Verification items for the finished model (mm, model axes). A direction names the side the tool comes from. Give positions to 0.01 mm unless a question says otherwise; leave off trailing zeros. Loops run counter-clockwise (first coordinate to the right, second up) from the corner with the lowest first, then second, coordinate; pieces in that order, holes last. Notation, with made-up numbers: (65.25, -21.75) -> (109.25, -21.75) arc R13 cw to (109.25, -17.75) -> close; hole circle Ø8 at (84.25, 73.5). An arc over 180 degrees is marked (long way). Answer in a Markdown table with one row per item. Add a question column.
Q1. Material ranges on probe 1 along Y at (x, z) = (-8.5, -10.5); probe 2 along Z at (x, y) = (-3.75, 3.75); probe 3 along Z at (x, y) = (13.25, 1.5), recorded low to high.
Q2. Section check C-C on x = -4. Enter the section's corners in (y, z), and give its area (3 significant figures).
Q3. Release check for a two-part mould opening along Z. For faces 1 (the face through (8, 1.8, -9)), 2 (the face through (0, 2.54, 8)), 3 (the face through (-6, 1, 7.562)) record: pulls with the +Z half, pulls with the -Z half, needs draft (parallel to the pull), parting line crosses it, or undercut.
Q4. Gauge pin test, flat ends, axial feed: P1, Ø1.5, axis at x = 11, y = 1.5, coming from the -Z side; P2, Ø2, axis at y = 1, z = 7.5, coming from the +X side; P3, Ø2, axis at x = -8.5, y = 0.5, coming from the +Z side; P4, Ø1, axis at x = -2.5, z = 9, coming from the +Y side. Record the tip position at first contact, or that the pin passes through.
Q5. Section check D-D on y = 0.75. Enter the section's corners in (x, z).
Q6. Section check B-B on z = -16. Enter the section's corners in (x, y).
Q7. Section check A-A on y = 3. Enter the section's corners in (x, z), and give its area (3 significant figures).
Q8. Set-up check for faces 4 (the face through (0, 6.88, -17)), 5 (the face through (11, 1, 5)), 6 (the face through (11, 1, -11)): record each of +Z, -Z, +X, -X, +Y, -Y from which the full face is reachable in a straight line by a thin tool's end or side.
```python
from build123d import *

# Parameters (mm, degrees)
SKETCH1_W           = 22
SKETCH1_H           = 28.216692514
BOSS_EXTRUDE1_DEPTH = 1.8
BOSS_EXTRUDE4_DEPTH = 2.54
SKETCH2_W           = 5.08
SKETCH2_H           = 5.08
BOSS_EXTRUDE2_DEPTH = 0.79375
BOSS_EXTRUDE3_START = -1.8
SKETCH3_W           = 7.62
SKETCH3_H           = 2.54
SKETCH3_W_2         = 20.32
SKETCH3_H_2         = 5.08
BOSS_EXTRUDE3_DEPTH = 5.08


with BuildPart() as part:
    # Sketch1 → Boss-Extrude1 (new body)
    with BuildSketch(Plane(origin=(0, 0, 0), x_dir=(1, 0, 0), z_dir=(0, 1, 0))):
        with Locations((0, 6.545846257)):
            Rectangle(SKETCH1_W, SKETCH1_H)
    extrude(amount=BOSS_EXTRUDE1_DEPTH)

    # Sketch4 → Boss-Extrude4 (add)
    with BuildSketch(Plane(origin=(0, 0, 0), x_dir=(1, 0, 0), z_dir=(0, 1, 0))):
        Polygon((-14.2875, -1.5875), (-1.5875, -1.5875), (-1.5875, -14.2875), (1.5875, -14.2875), (1.5875, -1.5875), (14.2875, -1.5875), (14.2875, 1.5875), (5, 1.5875), (5, 26.9875), (-5, 26.9875), (-5, 1.5875), (-14.2875, 1.5875), align=None)
    extrude(amount=BOSS_EXTRUDE4_DEPTH)

    # Sketch2 → Boss-Extrude2 (add)
    with BuildSketch(Plane(origin=(0, 1.8, 0), x_dir=(1, 0, 0), z_dir=(0, 1, 0))):
        Rectangle(SKETCH2_W, SKETCH2_H)
    extrude(amount=BOSS_EXTRUDE2_DEPTH)

    # Sketch3 → Boss-Extrude3 (add)
    with BuildSketch(Plane(origin=(0, 0, 0), x_dir=(-1, 0, 0), z_dir=(0, -1, 0)).offset(BOSS_EXTRUDE3_START)):
        with Locations((-1.27, 10.924192514)):
            Rectangle(SKETCH3_W, SKETCH3_H)
        with Locations((0, 17.274192514)):
            Rectangle(SKETCH3_W_2, SKETCH3_H_2)
    extrude(amount=-BOSS_EXTRUDE3_DEPTH)


solid = part.part
```
Taken from the geometry:
| question | item | result |
|---|---|---|
| 1 | probe 1 | y = 0 to 1.8 |
| 1 | probe 2 | z = -19.81 to -14.73 |
| 1 | probe 3 | z = -1.59 to 1.59 |
| 2 | outline | (0, -26.99) -> (2.54, -26.99) -> (2.54, -19.81) -> (6.88, -19.81) -> (6.88, -14.73) -> (2.54, -14.73) -> (2.54, 1.59) -> (1.8, 1.59) -> (1.8, 7.56) -> (0, 7.56) -> close |
| 2 | area | 105 mm² |
| 3 | face 1 | undercut |
| 3 | face 2 | needs draft |
| 3 | face 3 | pulls with the +Z half |
| 4 | P1 | stops at z = -20.65 |
| 4 | P2 | stops at x = 11 |
| 4 | P3 | stops at z = 7.56 |
| 4 | P4 | passes through |
| 5 | outline | (-14.29, -1.59) -> (-11, -1.59) -> (-11, -20.65) -> (-5, -20.65) -> (-5, -26.99) -> (5, -26.99) -> (5, -20.65) -> (11, -20.65) -> (11, -1.59) -> (14.29, -1.59) -> (14.29, 1.59) -> (11, 1.59) -> (11, 7.56) -> (1.59, 7.56) -> (1.59, 14.29) -> (-1.59, 14.29) -> (-1.59, 7.56) -> (-11, 7.56) -> (-11, 1.59) -> (-14.29, 1.59) -> close |
| 6 | outline | (-11, 0) -> (11, 0) -> (11, 1.8) -> (10.16, 1.8) -> (10.16, 6.88) -> (-10.16, 6.88) -> (-10.16, 1.8) -> (-11, 1.8) -> close |
| 7 | outline | (-10.16, -19.81) -> (10.16, -19.81) -> (10.16, -14.73) -> (-10.16, -14.73) -> close; (-2.54, -12.19) -> (5.08, -12.19) -> (5.08, -9.65) -> (-2.54, -9.65) -> close |
| 7 | area | 123 mm² |
| 8 | face 4 | +Z, -Z, +X, -X, +Y |
| 8 | face 5 | +Z, +X, +Y, -Y |
| 8 | face 6 | -Z, +X, +Y, -Y |
